from build123d import *

# Parameters (mm, degrees)
SKETCH1_R               = 5.5
SKETCH1_R_2             = 3.5
BOSS_EXTRUDE1_DEPTH     = 10
SKETCH2_R               = 2.5
BOSS_EXTRUDE2_DEPTH     = 170
SKETCH3_R               = 3.5
CUT_EXTRUDE1_DEPTH      = 11
BOSS_EXTRUDE3_DEPTH     = 5
SKETCH5_R               = 1.5
CUT_EXTRUDE2_DEPTH      = 7.5
CUT_EXTRUDE2_DEPTH_BACK = 5


with BuildPart() as part:
    # Sketch1 → Boss-Extrude1 (new body)
    with BuildSketch(Plane.XY):
        Circle(SKETCH1_R)
        Circle(SKETCH1_R_2, mode=Mode.SUBTRACT)
    extrude(amount=BOSS_EXTRUDE1_DEPTH)

    # Sketch2 → Boss-Extrude2 (add)
    with BuildSketch(Plane(origin=(0, 0, 0), x_dir=(1, 0, 0), z_dir=(0, 1, 0))):
        with Locations((0, -5)):
            Circle(SKETCH2_R)
    extrude(amount=BOSS_EXTRUDE2_DEPTH)

    # Sketch3 → Cut-Extrude1 (cut, through all)
    with BuildSketch(Plane.XY.offset(10)):
        Circle(SKETCH3_R)
    extrude(amount=-CUT_EXTRUDE1_DEPTH, mode=Mode.SUBTRACT)

    # Sketch4 → Boss-Extrude3 (add)
    with BuildSketch(Plane(origin=(0, 170, 0), x_dir=(1, 0, 0), z_dir=(0, 1, 0))):
        with BuildLine():
            Line((1, -7.291288), (1, -2.708712))
            ThreePointArc((1, -2.708712), (2.5, -5), (1, -7.291288))
        make_face()
        with BuildLine():
            Line((-1, -7.291288), (-1, -2.708712))
            ThreePointArc((-1, -2.708712), (-2.5, -5), (-1, -7.291288))
        make_face()
    extrude(amount=BOSS_EXTRUDE3_DEPTH)

    # Sketch5 → Cut-Extrude2 (cut, two sides)
    with BuildSketch(Plane(origin=(-1, 0, 0), x_dir=(0, 0, -1), z_dir=(1, 0, 0))) as cut_extrude2_sk:
        with Locations((-4.791288, 172.5)):
            Circle(SKETCH5_R)
    extrude(amount=CUT_EXTRUDE2_DEPTH, mode=Mode.SUBTRACT)
    extrude(cut_extrude2_sk.sketch, amount=-CUT_EXTRUDE2_DEPTH_BACK, mode=Mode.SUBTRACT)


solid = part.part
Can you work these out from the model? Positions are in its coordinate system, mm. A direction names the side the tool comes from. Coordinates: 2 decimals unless noted, no trailing zeros. Write each loop counter-clockwise with the first axis right and the second up, starting at its lowest first coordinate (ties: lowest second). Pieces come first, ordered by that corner, then holes. Notation, with made-up numbers: (-4, 89.5) -> (37, 89.5) arc R10 ccw to (37, 106.5) -> close; hole circle Ø3 at (-27, 68). An arc over 180 degrees is marked (long way). Write item = value, one per line.
(1) Imagine slicing it at C-C (y = 97.5). Please give me the cut outline in (x, z), and give its area (3 significant figures).
Verdict:
outline = circle Ø5 at (0, 5)
area = 19.6 mm^2
(2) Imagine slicing it at B-B (y = 0). Please give me the cut outline in (x, z), and give its area (3 significant figures).
Verdict:
outline = (-5.5, 0) -> (-3.5, 0) -> (-3.5, 10) -> (-5.5, 10) -> close; (3.5, 0) -> (5.5, 0) -> (5.5, 10) -> (3.5, 10) -> close
area = 40.0 mm^2
(3) Imagine slicing it at A-A (y = 172.5). Please give me the cut outline in (x, z), and give its area (3 significant figures).
Verdict:
outline = (-2.14, 6.29) -> (-1, 6.29) -> (-1, 7.29) arc R2.5 ccw to start; (-1.82, 3.29) arc R2.5 ccw to (-1, 2.71) -> (-1, 3.29) -> close; (1, 2.71) arc R2.5 ccw to (1.82, 3.29) -> (1, 3.29) -> close; (1, 6.29) -> (2.14, 6.29) arc R2.5 ccw to (1, 7.29) -> close
area = 1.93 mm^2
(4) If I drill on probe 1 along Y at (x, z) = (-0.25, 5.75); probe 2 along Y at (x, z) = (-1.25, 3.5); probe 3 along Y at (x, z) = (-0.25, 1.75), over which ranges is the centre line in solid material (lowest first)?
Verdict:
probe_1 = -5.49 to -3.49, 3.49 to 170
probe_2 = -5.36 to -3.27, 3.27 to 171.74, 173.26 to 175
probe_3 = -5.49 to -3.49, 3.49 to 5.49
(5) Thinking about a two-plate mould opening in Y: for faces 3 (the face through (1, 172, 7)), 4 (the face through (-1.57, 172.57, 6.29)), 5 (the face through (-1.19, -5.37, 4.93)), which applies, +Y half, -Y half, draft (parallel to the pull), parting line (faces both ways), or undercut?
Verdict:
face_3 = draft
face_4 = undercut
face_5 = parting line
(6) For pin 1 (1 mm diameter, centred on y = 146, z = 6.5, fed in from +X); pin 2 (1 mm diameter, centred on x = 0, y = 106.5, fed in from -Z); pin 3 (0.6 mm diameter, centred on x = 0, z = 4, fed in from +Y), each with a flat end and sliding along its axis, tell me the tip position at first contact or that it passes through.
Verdict:
pin_1 = 2.29
pin_2 = 2.5
pin_3 = 170
(7) On a 3-axis mill with a long thin cutter (end or side, diameter ignored), from which of +Z, -Z, +X, -X, +Y, -Y can I reach the whole of each face in a straight line? I mean faces 1 (the face through (-1, 172, 7)), 2 (the face through (1.57, 172.57, 6.29)). Say none if no direction works.
Verdict:
face_1 = +Z, -Z, +Y
face_2 = +X, -X
